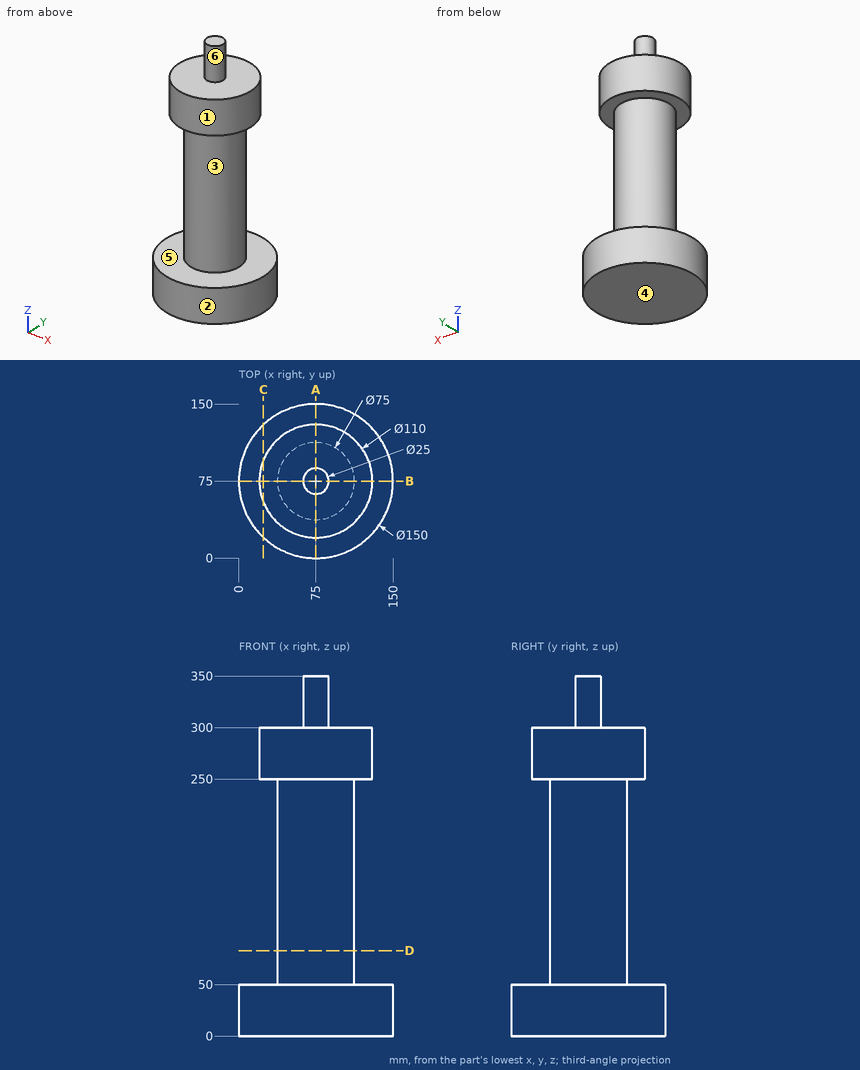
Design review of the part shown in the three views and the two pictorial views. Dimensions are in mm from the part's minimum x, y and z. A direction names the side the tool comes from. Give positions to 0.01 mm unless a question says otherwise; leave off trailing zeros. Loops run counter-clockwise (first coordinate to the right, second up) from the corner with the lowest first, then second, coordinate; pieces in that order, holes last. Notation, with made-up numbers: (13.5, 38) -> (39.5, 38) arc R22 cw to (39.5, 71) -> close; hole circle Ø10 at (11, 19.5). An arc over 180 degrees is marked (long way). Write each question's results on one line, items separated by ' | '.
Q1. Machinability: for the marked faces 1, 2 and 3, which of the approach directions +Z, -Z, +X, -X, +Y, -Y give a long, thin tool a straight path to every point of the face, cutting with its end or side? Answer none if there is none.
Reply:
face 1: +Z | face 2: +Z, -Z | face 3: none
Q2. Wall thickness on L1, parallel to Z at x = 26.5, y = 91; L2, parallel to Z at x = 106, y = 139; L3, parallel to Z at x = 93.5, y = 59: over which ranges is each line inside the solid? List them lowest first.
Reply:
L1: z = 0 to 50, 250 to 300 | L2: z = 0 to 50 | L3: z = 0 to 300
Q3. Take a section at C-C, the plane x = 24. Write out the cut boundary in (y, z), plus the area to 3 significant figures.
Reply:
outline: (20.01, 0) -> (129.99, 0) -> (129.99, 50) -> (20.01, 50) -> close; (54.41, 250) -> (95.59, 250) -> (95.59, 300) -> (54.41, 300) -> close | area: 7,560 mm²
Q4. Take a section at A-A, the plane x = 75. Write out the cut boundary in (y, z).
Reply:
outline: (0, 0) -> (150, 0) -> (150, 50) -> (112.5, 50) -> (112.5, 250) -> (130, 250) -> (130, 300) -> (87.5, 300) -> (87.5, 350) -> (62.5, 350) -> (62.5, 300) -> (20, 300) -> (20, 250) -> (37.5, 250) -> (37.5, 50) -> (0, 50) -> close
Q5. For pin 1 Ø1 at (x, y) = (91.5, 55.5) entering from +Z; pin 2 Ø12 at (x, z) = (103.5, 76) entering from -Y; pin 3 Ø12 at (y, z) = (94.5, 235) entering from +X, all flat-tipped, find the tip position at first contact; note any pin that passes through.
Reply:
pin 1: stops at z = 300 | pin 2: stops at y = 45 | pin 3: stops at x = 109.99
Q6. The part is to be moulded in two halves that separate along Z. For the marked faces 4, 5 and 6, say which applies: +Z half, -Z half, draft (parallel to the pull), parting line (faces both ways), or undercut.
Reply:
face 4: -Z half | face 5: undercut | face 6: draft
Q7. Take a section at D-D, the plane z = 83. Write out the cut boundary in (x, y).
Reply:
outline: circle Ø75 at (75, 75)
